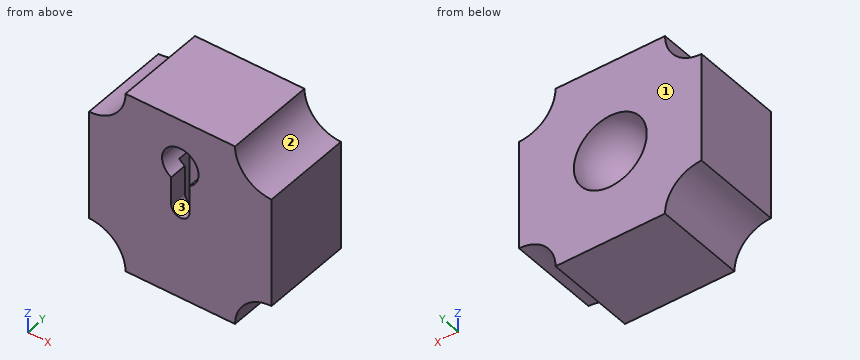
```python
from build123d import *

# Parameters (mm, degrees)
SKETCH1_W           = 50
SKETCH1_H           = 50
BOSS_EXTRUDE1_DEPTH = 25
SKETCH2_R           = 10
CUT_EXTRUDE1_DEPTH  = 25
CUT_EXTRUDE6_DEPTH  = 8.6
CUT_EXTRUDE8_START  = -8
CUT_EXTRUDE8_DEPTH  = 24


with BuildPart() as part:
    # Sketch1 → Boss-Extrude1 (new body)
    with BuildSketch(Plane(origin=(0, 0, 0), x_dir=(1, 0, 0), z_dir=(0, 1, 0))):
        Rectangle(SKETCH1_W, SKETCH1_H)
    extrude(amount=BOSS_EXTRUDE1_DEPTH)

    # Sketch2 → Cut-Extrude1 (cut)
    with BuildSketch(Plane(origin=(0, 25, 0), x_dir=(1, 0, 0), z_dir=(0, 1, 0))):
        with Locations((-25, -25)):
            Circle(SKETCH2_R)
        with Locations((-25, 25)):
            Circle(SKETCH2_R)
        with Locations((25, 25)):
            Circle(SKETCH2_R)
        with Locations((25, -25)):
            Circle(SKETCH2_R)
    extrude(amount=-CUT_EXTRUDE1_DEPTH, mode=Mode.SUBTRACT)

    # Sketch3 → Cut-Revolve1 (revolve, cut)
    with BuildSketch(Plane(origin=(0, 25, 0), x_dir=(1, 0, 0), z_dir=(0, 1, 0))):
        with BuildLine():
            Line((0, 10), (0, -10))
            ThreePointArc((0, -10), (-10, 0), (0, 10))
        make_face()
    revolve(axis=Axis((0, 25, -10), (0, 0, 1)), mode=Mode.SUBTRACT)

    # Sketch4 → Cut-Extrude6 (cut)
    with BuildSketch(Plane(origin=(0, 0, 0), x_dir=(-1, 0, 0), z_dir=(0, -1, 0))):
        with BuildLine():
            ThreePointArc((2.5, 0), (0, 2.5), (-2.5, 0))
            Line((-2.5, 0), (2.5, 0))
        make_face()
        with BuildLine():
            Line((2.5, 0), (-2.5, 0))
            ThreePointArc((-2.5, 0), (0, -2.5), (2.5, 0))
        make_face()
        with BuildLine():
            ThreePointArc((2.5, 0), (0, -2.5), (-2.5, 0))
            Line((-2.5, 0), (-2.5, -7.669872981))
            ThreePointArc((-2.5, -7.669872981), (0, -7), (2.5, -7.669872981))
            Line((2.5, -7.669872981), (2.5, 0))
        make_face()
        with BuildLine():
            ThreePointArc((2.5, -7.669872981), (0, -7), (-2.5, -7.669872981))
            Line((-2.5, -7.669872981), (2.5, -7.669872981))
        make_face()
        with BuildLine():
            Line((2.5, -7.669872981), (-2.5, -7.669872981))
            ThreePointArc((-2.5, -7.669872981), (-2.5, -16.330127019), (5, -12))
            ThreePointArc((5, -12), (4.330127019, -9.5), (2.5, -7.669872981))
        make_face()
    extrude(amount=-CUT_EXTRUDE6_DEPTH, mode=Mode.SUBTRACT)

    # Sketch5 → Cut-Extrude8 (cut)
    with BuildSketch(Plane.XY.offset(25).offset(CUT_EXTRUDE8_START)):
        Polygon((0, 4.9), (-4, 4.9), (-4, 8.6), (4, 8.6), (4, 4.9), align=None)
    extrude(amount=-CUT_EXTRUDE8_DEPTH, mode=Mode.SUBTRACT)


solid = part.part
```
Build history of the part. All positions in model axes, mm. Face numbers are marked on the shaded views. Give positions to 0.01 mm unless a question says otherwise; leave off trailing zeros. Loops run counter-clockwise (first coordinate to the right, second up) from the corner with the lowest first, then second, coordinate; pieces in that order, holes last.
1) Probe line 1 along Z through (x, y) = (0, 3.25); line 2 along Z through (x, y) = (-2, 6.5); line 3 along X through (y, z) = (3.25, 12). List the from-to ranges inside material, lowest first.
Values follow:
line 1: z = -25 to -2.5, 17 to 25
line 2: z = -25 to -7, 17 to 25
line 3: x = -25 to -5, 5 to 25
2) Drop flat-ended pins along their axis: P1, Ø3, axis at x = 1, z = 8, coming from the -Y side; P2, Ø1.5, axis at x = 3, z = -5, coming from the +Y side; P3, Ø0.6, axis at y = 6.5, z = 16.5, coming from the -X side. Give the stop position or say it passes through.
Values follow:
P1: stops at y = 8.6
P2: stops at y = 17.47
P3: stops at x = -20.25
3) Band-saw the part on B-B on x = -6. List the corners of the cut face in (y, z).
Values follow:
outline: (0, -25) - (25, -25) - (25, -8) arc R8 cw to (25, 8) - (25, 25) - (0, 25) - close
4) Band-saw the part on D-D on z = -5. List the corners of the cut face in (x, y), then the cut area to 3 significant figures.
Values follow:
outline: (-25, 0) - (25, 0) - (25, 25) - (8.66, 25) arc R8.66 cw to (-8.66, 25) - (-25, 25) - close; hole (-4, 4.9) - (4, 4.9) - (4, 8.6) - (-4, 8.6) - close
area: 1,100 mm2
5) Band-saw the part on C-C on y = 12. List the corners of the cut face in (x, z).
Values follow:
outline: (-25, -15) arc R10 cw to (-15, -25) - (15, -25) arc R10 cw to (25, -15) - (25, 15) arc R10 cw to (15, 25) - (-15, 25) arc R10 cw to (-25, 15) - close
6) Band-saw the part on A-A on y = 17. List the corners of the cut face in (x, z), then the cut area to 3 significant figures.
Values follow:
outline: (-25, -15) arc R10 cw to (-15, -25) - (15, -25) arc R10 cw to (25, -15) - (25, 15) arc R10 cw to (15, 25) - (-15, 25) arc R10 cw to (-25, 15) - close; hole circle Ø12 at (0, 0)
area: 2,070 mm2
7) Two-plate mould, pull along Z, no slides. Class the marked faces 1, 2 and 3: released by +Z, released by -Z, zero draft, split by the parting line, or undercut.
Values follow:
face 1: zero draft
face 2: released by +Z
face 3: undercut
